```python
from build123d import *

# Parameters (mm, degrees)
SKETCH1_R           = 70.8759
SKETCH1_R_2         = 1.4732
SKETCH1_R_3         = 40
BOSS_EXTRUDE1_DEPTH = 1.6
SKETCH1_3_R         = 65
SKETCH1_3_R_2       = 57
CUT_EXTRUDE1_DEPTH  = 0.1


with BuildPart() as part:
    # Sketch1 → Boss-Extrude1 (new body)
    with BuildSketch(Plane(origin=(0, 0, 0), x_dir=(1, 0, 0), z_dir=(0, 1, 0))):
        with Locations(Location((0, 0, 0), (0, 0, 270))):
            Circle(SKETCH1_R)
        with Locations(Location((0, 67.93795, 0), (0, 0, 270))):
            Circle(SKETCH1_R_2, mode=Mode.SUBTRACT)
        with Locations(Location((58.835990581, 33.968975, 0), (0, 0, 270))):
            Circle(SKETCH1_R_2, mode=Mode.SUBTRACT)
        with Locations(Location((58.835990581, -33.968975, 0), (0, 0, 270))):
            Circle(SKETCH1_R_2, mode=Mode.SUBTRACT)
        with Locations(Location((0, -67.93795, 0), (0, 0, 270))):
            Circle(SKETCH1_R_2, mode=Mode.SUBTRACT)
        with Locations(Location((-58.835990581, -33.968975, 0), (0, 0, 270))):
            Circle(SKETCH1_R_2, mode=Mode.SUBTRACT)
        with Locations(Location((-58.835990581, 33.968975, 0), (0, 0, 270))):
            Circle(SKETCH1_R_2, mode=Mode.SUBTRACT)
        with Locations(Location((0, 0, 0), (0, 0, 270))):
            Circle(SKETCH1_R_3, mode=Mode.SUBTRACT)
        with Locations(Location((0, 48.5, 0), (0, 0, 270))):
            Circle(SKETCH1_R_2, mode=Mode.SUBTRACT)
        with Locations(Location((42.002232084, 24.25, 0), (0, 0, 270))):
            Circle(SKETCH1_R_2, mode=Mode.SUBTRACT)
        with Locations(Location((42.002232084, -24.25, 0), (0, 0, 270))):
            Circle(SKETCH1_R_2, mode=Mode.SUBTRACT)
        with Locations(Location((0, -48.5, 0), (0, 0, 270))):
            Circle(SKETCH1_R_2, mode=Mode.SUBTRACT)
        with Locations(Location((-42.002232084, -24.25, 0), (0, 0, 270))):
            Circle(SKETCH1_R_2, mode=Mode.SUBTRACT)
        with Locations(Location((-42.002232084, 24.25, 0), (0, 0, 270))):
            Circle(SKETCH1_R_2, mode=Mode.SUBTRACT)
    extrude(amount=BOSS_EXTRUDE1_DEPTH)

    # Sketch1_3 → Cut-Extrude1 (cut)
    with BuildSketch(Plane(origin=(0, 0, 0), x_dir=(1, 0, 0), z_dir=(0, 1, 0))):
        with Locations(Location((0, 0, 0), (0, 0, 270))):
            Circle(SKETCH1_3_R)
        with Locations(Location((0, 0, 0), (0, 0, 270))):
            Circle(SKETCH1_3_R_2, mode=Mode.SUBTRACT)
    extrude(amount=CUT_EXTRUDE1_DEPTH, mode=Mode.SUBTRACT)


solid = part.part
```
Model file for the job. Use its own axes, mm. Give positions to 0.01 mm unless a question says otherwise; leave off trailing zeros. Write each loop counter-clockwise with the first axis right and the second up, starting at its lowest first coordinate (ties: lowest second). Pieces come first, ordered by that corner, then holes. Notation, with made-up numbers: (7, -16.5) - (13, -16.5) arc R13 cw to (13, -5.5) - close; hole circle Ø4 at (89.25, -11). An arc over 180 degrees is marked (long way). One line per question, with ' | ' between items. Start each with the question number.
(1) Slice it at D-D on x = 62.5. Write the cut outline in (y, z), plus the area to 3 significant figures.
(2) Two-plate mould, pull along X, no slides. Class faces 1 (the face through (-12, 0, -39)), 2 (the face through (-39.05, 0.79, -8.67)), 3 (the face through (3.116, 0.789, -70.807)): +X half, -X half, draft (parallel to the pull), parting line (faces both ways), or undercut.
(3) Slice it at A-A on z = 0. Write the cut outline in (x, y), plus the area to 3 significant figures.
(4) Wall check: line 1 along X through (y, z) = (0.8, -25.5); line 2 along Z through (x, y) = (-43, 1.3); line 3 along X through (y, z) = (1, 3.5). Give the ranges that are in metal, low to high. Write a range as from..to.
(5) Pin check, flat tips, straight feed: P1, Ø4, axis at x = -42, z = -24.25, coming from the +Y side; P2, Ø1.8, axis at x = -58.84, z = 33.97, coming from the +Y side. Stop position of each tip, or through.
(6) Slice it at C-C on z = 18.5. Write the cut outline in (x, y), plus the area to 3 significant figures.
(7) Slice it at B-B on y = 0.45. Give the number of separate pieces and of enclosed holes in the cut face, plus the area to 3 significant figures.
Results below:
1) outline: (0, -33.42) - (1.6, -33.42) - (1.6, 33.42) - (0, 33.42) - (0, 17.85) - (0.1, 17.85) - (0.1, -17.85) - (0, -17.85) - close | area: 103 mm^2
2) face 1: draft | face 2: undercut | face 3: parting line
3) outline: (-70.88, 0) - (-65, 0) - (-65, 0.1) - (-57, 0.1) - (-57, 0) - (-40, 0) - (-40, 1.6) - (-70.88, 1.6) - close; (40, 0) - (57, 0) - (57, 0.1) - (65, 0.1) - (65, 0) - (70.88, 0) - (70.88, 1.6) - (40, 1.6) - close | area: 97.2 mm^2
4) line 1: -66.13..-42.78, -41.22..-30.82, 30.82..41.22, 42.78..66.13 | line 2: -56.34..-25.33, -23.17..23.17, 25.33..56.34 | line 3: -70.79..-39.85, 39.85..70.79
5) P1: y = 1.6 | P2: through
6) outline: (-68.42, 0) - (-62.31, 0) - (-62.31, 0.1) - (-53.91, 0.1) - (-53.91, 0) - (-35.46, 0) - (-35.46, 1.6) - (-68.42, 1.6) - close; (35.46, 0) - (53.91, 0) - (53.91, 0.1) - (62.31, 0.1) - (62.31, 0) - (68.42, 0) - (68.42, 1.6) - (35.46, 1.6) - close | area: 104 mm^2
7) separate pieces: 1 | enclosed holes: 13 | area: 10,700 mm^2
